The model under review builds one solid part; all positions refer to its coordinate system, in mm. Round coordinates to 2 decimals unless told otherwise and drop trailing zeros. Order: outer loops, then holes, each group sorted by start corner. A loop starts at its lowest first (then second) coordinate and runs counter-clockwise, first axis right, second up. Notation, with made-up numbers: M -23,86 L 3,86 A20 cw 3,95 Z; hole C 27,54 d2. An arc over 180 degrees is marked long. Answer as a JSON object with one key per item and string values. Group by question number.
1) The part is to be moulded in two halves that separate along Z. For faces 1 (the flat face through (-13, 6.35, -25)), 2 (the flat face through (-13, 3, -50.8)), 3 (the cylindrical face through (-5.7, 3.13, -10.65)), say which applies: +Z half, -Z half, draft (parallel to the pull), parting line (faces both ways), or undercut.
2) Insertion check: pin 1 Ø3.5 at (x, z) = (-21.59, -40.4) entering from +Y. The pin has a flat end and moves straight along its axis. Give the tip position at first contact, or say it passes through.
3) Consider section A-A, the plane x = -3.81. Write out the cut boundary in (y, z), then the cut area to 3 significant figures.
4) To check wall thickness, follow line 1 (Z direction, x = -3.81, y = 2); line 2 (X direction, y = 5.5, z = -11); line 3 (X direction, y = 2.5, z = -39.5). State the ranges of each line that lie inside material, in increasing order.
5) Consider section B-B, the plane y = 2.5. Write out the cut boundary in (x, z) (3 decimals).
Autodesk Inventor part; units mm, degrees
ref_plane "YZ Plane" through (0, 0, 0) normal (1, 0, 0) x (0, 1, 0)
ref_plane "XZ Plane" through (0, 0, 0) normal (0, 1, 0) x (-1, 0, 0)
ref_plane "XY Plane" through (0, 0, 0) normal (0, 0, 1) x (1, 0, 0)
sketch "Sketch1" plane through (0, 0, 0) normal (0, 1, 0) x (-1, 0, 0)
  line L0 (0, 0) -> (25.4, 0)
  line L1 (25.4, 0) -> (25.4, -50.8)
  line L2 (25.4, -50.8) -> (0, -50.8)
  line L3 (0, -50.8) -> (0, 0)
  dimension "d0" = 50.8
  dimension "d1" = 25.4
extrude "Extrusion1" add sketch "Sketch1" along normal blind 6.35
sketch "Sketch2" plane through (0, 6.35, 0) normal (0, 1, 0) x (1, 0, 0)
  line L0 (-25.4, 0) -> (0, 0)
  line L1 (0, 0) -> (0, 50.8)
  line L2 (0, 50.8) -> (-25.4, 50.8)
  line L3 (-25.4, 50.8) -> (-25.4, 0)
  point P0 (-21.59, 10.4013)
  point P1 (-21.59, 40.3987)
  point P2 (-3.81, 10.4013)
  point P3 (-3.81, 40.3987)
  dimension "d4" = 29.9974
  dimension "d5" = 50.8
  dimension "d6" = 10.4013
  dimension "d9" = 29.9974
  dimension "d10" = 3.81
  dimension "d11" = 3.81
  dimension "d12" = 3.81
  dimension "d13" = 3.81
  dimension "d14" = 10.4013
hole "Hole1" at (-21.59, 6.35, -10.4013) at (-21.59, 6.35, -40.3987) at (-3.81, 6.35, -10.4013) at (-3.81, 6.35, -40.3987) direction (0, -1, 0) diameter 3.81 depth 25.4 tip angle 118
properties part number "20X20 carege"
Results list:
{
 "1": {"face 1": "draft", "face 2": "-Z half", "face 3": "undercut"},
 "2": {"pin 1": "through"},
 "3": {"outline": "M 0,-50.8 L 6.35,-50.8 L 6.35,-42.3 L 0,-42.3 Z; M 0,-38.49 L 6.35,-38.49 L 6.35,-12.31 L 0,-12.31 Z; M 0,-8.5 L 6.35,-8.5 L 6.35,0 L 0,0 Z", "area": "274 mm^2"},
 "4": {"line 1": "-50.8 to -42.3, -38.49 to -12.31, -8.5 to 0", "line 2": "-25.4 to -23.4, -19.78 to -5.62, -2 to 0", "line 3": "-25.4 to -23.27, -19.91 to -5.49, -2.13 to 0"},
 "5": {"outline": "M -25.4,-50.8 L 0,-50.8 L 0,0 L -25.4,0 Z; hole C -21.59,-40.399 d3.81; hole C -21.59,-10.401 d3.81; hole C -3.81,-40.399 d3.81; hole C -3.81,-10.401 d3.81"}
}
